Input: part model. Units: mm. Frame: model coordinates. Coordinates: 2 decimals unless noted, no trailing zeros. Order: outer loops, then holes, each group sorted by start corner. A loop starts at its lowest first (then second) coordinate and runs counter-clockwise, first axis right, second up. Notation, with made-up numbers: (69.5, 38) - (113.5, 38) arc R28 cw to (113.5, 75) - close; hole circle Ø8 at (87, 62). An arc over 180 degrees is marked (long way). One line per question, with ' | ' between items. Start each with the question number.
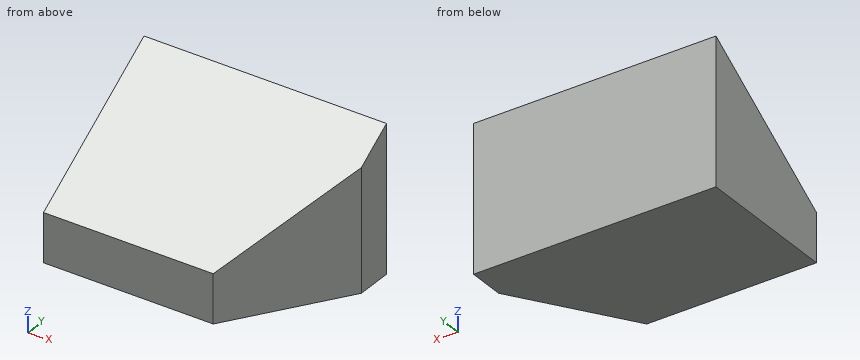
```python
from build123d import *

# Parameters (mm, degrees)
F0_W     = 100
F0_H     = 60
F1_DEPTH = 60
F3_DEPTH = 60
F5_DEPTH = 100


with BuildPart() as f1:
    # F0 (on Top) → F1 (new body)
    with BuildSketch(Plane.XY):
        with Locations((50, -30)):
            Rectangle(F0_W, F0_H)
    extrude(amount=F1_DEPTH)

    # F2 (on face) → F3 (cut, through all)
    with BuildSketch(Plane.XY.offset(60)):
        Polygon((100, -60), (100, -15), (70, -60), align=None)
    extrude(amount=-F3_DEPTH, mode=Mode.SUBTRACT)

    # F4 (on face) → F5 (cut, through all)
    with BuildSketch(Plane(origin=(0, 0, 0), x_dir=(0, -1, 0), z_dir=(-1, 0, 0))):
        Polygon((60, 60), (0, 60), (60, 20), align=None)
    extrude(amount=-F5_DEPTH, mode=Mode.SUBTRACT)


solid = f1.part
```
(1) Section B-B (y = -12). Output: boundary loops of the cut face in (x, z), then the cut area to 3 significant figures.
(2) Section A-A (z = 5.5). Output: boundary loops of the cut face in (x, y).
(3) Material intervals for line 1 along Y through (x, z) = (78, 12); line 2 along Y through (x, z) = (30, 32); line 3 along X through (y, z) = (-20, 17), sorted ascending. Write a range as from..to.
(4) Section C-C (x = 90). Output: boundary loops of the cut face in (y, z).
(5) Pin query (flat end, axial travel): pin 1 (6 mm diameter, centred on x = 80.5, z = 27.5, fed in from -Y); pin 2 (12 mm diameter, centred on y = -36, z = 20.5, fed in from +X); pin 3 (2 mm diameter, centred on x = 10.5, y = -11, fed in from +Z). Return the tip coordinate at first contact, or that it passes through.
(6) Section D-D (z = 21.5). Output: boundary loops of the cut face in (x, y), then the cut area to 3 significant figures.
Worked answers:
1) outline: (0, 0) - (100, 0) - (100, 52) - (0, 52) - close | area: 5,200 mm²
2) outline: (0, -60) - (70, -60) - (100, -15) - (100, 0) - (0, 0) - close
3) line 1: y = -48..0 | line 2: y = -42..0 | line 3: x = 0..96.67
4) outline: (-30, 0) - (0, 0) - (0, 60) - (-30, 40) - close
5) pin 1: stops at y = -48.75 | pin 2: stops at x = 90 | pin 3: stops at z = 53.33
6) outline: (0, -57.75) - (71.5, -57.75) - (100, -15) - (100, 0) - (0, 0) - close | area: 5,170 mm²
